Could you check a few things on this model? Use its own coordinates, in mm. Face numbers are marked on the shaded views. A direction names the side the tool comes from. Coordinates: 2 decimals unless noted, no trailing zeros. Order: outer loops, then holes, each group sorted by start corner. A loop starts at its lowest first (then second) coordinate and runs counter-clockwise, first axis right, second up. Notation, with made-up numbers: (-20.75, -33.75) - (9.25, -33.75) arc R22 cw to (9.25, -10.75) - close; hole circle Ø4 at (-33.75, 83). An arc over 180 degrees is marked (long way). Answer as CSV lines item,"result". Start each with the question number.
1. I want a section at B-B, the plane z = 0.55. Count the separate pieces of the cut face and the enclosed holes in it, and give its area (3 significant figures).
2. For the marked faces 1 and 2, which set-ups out of +Z, -Z, +X, -X, +Y, -Y let a thin tool reach every point of the face, with its end or its side?
3. For pin 1 (12 mm diameter, centred on x = 24.5, y = 22.5, fed in from +Z); pin 2 (1 mm diameter, centred on x = 20.5, z = 1, fed in from -Y); pin 3 (1.5 mm diameter, centred on x = 17.5, z = 3, fed in from -Y), each with a flat end and sliding along its axis, tell me the tip position at first contact or that it passes through.
4. I want a section at A-A, the plane x = 30. List the corners of the cut face in (y, z) for me.
5. I want a section at D-D, the plane x = 15.5. List the corners of the cut face in (y, z) for me.
6. I need wall thicknesses on probe 1 along Y at (x, z) = (30, 1.3); probe 2 along X at (y, z) = (15.5, 2.9); probe 3 along X at (y, z) = (37, 0.7). Which ranges of each line are inside material? Lowest first, please.
7. I want a section at C-C, the plane y = 16. List the corners of the cut face in (x, z) for me.
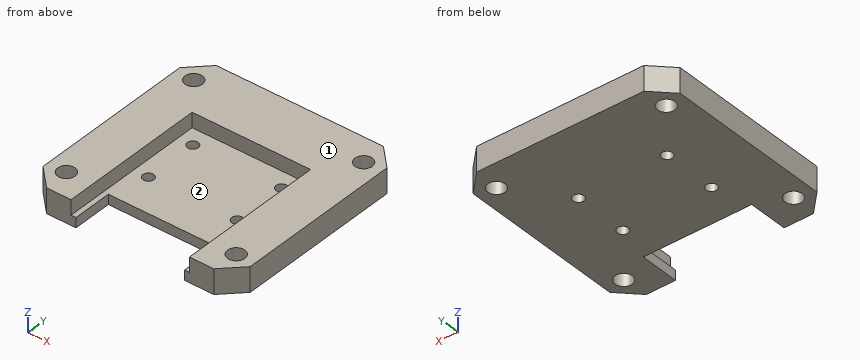
from build123d import *

# Parameters (mm, degrees)
SKETCH1_R               = 1.75
BOSS_EXTRUDE1_DEPTH     = 5
CUT_EXTRUDE1_DEPTH      = 60.607046563
CUT_EXTRUDE1_DEPTH_BACK = 60.607046563
SKETCH2_W               = 22
SKETCH2_H               = 8
SKETCH3_W               = 24
SKETCH3_H               = 30
CUT_EXTRUDE2_DEPTH      = 3
SKETCH4_R               = 1.1
CUT_EXTRUDE3_DEPTH      = 3


with BuildPart() as part:
    # Sketch1 → Boss-Extrude1 (new body)
    with BuildSketch(Plane.XY):
        Polygon((4.055, 42), (0, 37.945), (0, 4.055), (4.055, 0), (37.945, 0), (42, 4.055), (42, 37.945), (37.945, 42), align=None)
        with Locations((3.779747468, 36.775)):
            Circle(SKETCH1_R, mode=Mode.SUBTRACT)
        with Locations((3.779747468, 5.225)):
            Circle(SKETCH1_R, mode=Mode.SUBTRACT)
        with Locations(Location((38.220252532, 5.225, 0), (0, 0, 180))):
            Circle(SKETCH1_R, mode=Mode.SUBTRACT)
        with Locations(Location((38.220252532, 36.775, 0), (0, 0, 180))):
            Circle(SKETCH1_R, mode=Mode.SUBTRACT)
    extrude(amount=BOSS_EXTRUDE1_DEPTH)

    # Sketch2 → Cut-Extrude1 (cut, two sides: drawn at the far end of the back side and taken through both)
    with BuildSketch(Plane.XY.offset(5).offset(-CUT_EXTRUDE1_DEPTH_BACK)):
        with Locations((21, 4)):
            Rectangle(SKETCH2_W, SKETCH2_H)
    extrude(amount=CUT_EXTRUDE1_DEPTH + CUT_EXTRUDE1_DEPTH_BACK, mode=Mode.SUBTRACT)

    # Sketch3 → Cut-Extrude2 (cut)
    with BuildSketch(Plane.XY.offset(5)):
        with Locations((21, 15)):
            Rectangle(SKETCH3_W, SKETCH3_H)
    extrude(amount=-CUT_EXTRUDE2_DEPTH, mode=Mode.SUBTRACT)

    # Sketch4 → Cut-Extrude3 (cut)
    with BuildSketch(Plane.XY.offset(2)):
        with Locations((12, 26.5)):
            Circle(SKETCH4_R)
        with Locations((30, 26.5)):
            Circle(SKETCH4_R)
        with Locations((12, 15.5)):
            Circle(SKETCH4_R)
        with Locations((30, 15.5)):
            Circle(SKETCH4_R)
    extrude(amount=-CUT_EXTRUDE3_DEPTH, mode=Mode.SUBTRACT)


solid = part.part
Solved:
1,separate pieces,"1"
1,enclosed holes,"8"
1,area,"1,500 mm2"
2,face 1,"+Z, +X, -X, +Y, -Y"
2,face 2,"+Z, -Y"
3,pin 1,"stops at z = 2"
3,pin 2,"stops at y = 8"
3,pin 3,"stops at y = 30"
4,outline,"(8, 0) - (14.4, 0) - (14.4, 2) - (8, 2) - close; (16.6, 0) - (25.4, 0) - (25.4, 2) - (16.6, 2) - close; (27.6, 0) - (42, 0) - (42, 5) - (30, 5) - (30, 2) - (27.6, 2) - close"
5,outline,"(8, 0) - (42, 0) - (42, 5) - (30, 5) - (30, 2) - (8, 2) - close"
6,probe 1,"y = 8 to 14.4, 16.6 to 25.4, 27.6 to 42"
6,probe 2,"x = 0 to 9, 33 to 42"
6,probe 3,"x = 0 to 2.04, 5.52 to 36.48, 39.96 to 42"
7,outline,"(0, 0) - (11.02, 0) - (11.02, 2) - (9, 2) - (9, 5) - (0, 5) - close; (12.98, 0) - (29.02, 0) - (29.02, 2) - (12.98, 2) - close; (30.98, 0) - (42, 0) - (42, 5) - (33, 5) - (33, 2) - (30.98, 2) - close"
